Model file for the job. Use its own axes, mm. Face numbers are marked on the shaded views. Coordinates: 2 decimals unless noted, no trailing zeros. Write each loop counter-clockwise with the first axis right and the second up, starting at its lowest first coordinate (ties: lowest second). Pieces come first, ordered by that corner, then holes. Notation, with made-up numbers: (78.25, 63) - (137.25, 63) arc R22 cw to (137.25, 101) - close; hole circle Ø6 at (-8, -38). An arc over 180 degrees is marked (long way). Put each result on its own line as item: value. Start each with the question number.
1. Saw through at D-D, the plane x = 66. Write the cut outline in (y, z).
2. Pull direction X, two halves, no side cores. Call the marked faces 1, 2 and 3: released by +X, released by -X, zero draft, split by the parting line, or undercut.
3. Drill centre lines: L1, parallel to X at y = 7, z = -11; L2, parallel to X at y = 29, z = -8; L3, parallel to Z at x = 21, y = 13. Where is each one in solid material? Low to high. Write a range as from..to.
4. Drop a flat-ended pin along its axis: P1, Ø4, axis at x = -52.5, y = 15, coming from the -Z side. Give the stop position or say it passes through.
5. Saw through at A-A, the plane z = 15. Write the cut outline in (x, y).
6. Saw through at B-B, the plane x = -7. Write the cut outline in (y, z).
7. Saw through at C-C, the plane y = 8.5. Write the cut outline in (x, z), plus the area to 4 significant figures.
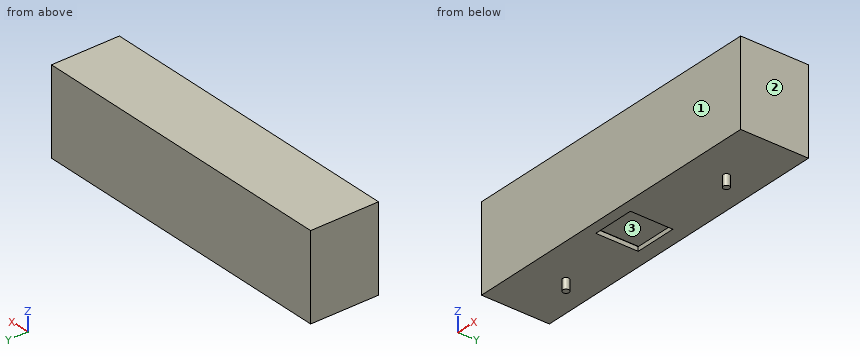
```python
from build123d import *

# Parameters (mm, degrees)
SKETCH1_W           = 150
SKETCH1_H           = 40
BOSS_EXTRUDE1_DEPTH = 30
SHELL3_T            = -2
SKETCH3_W           = 20
SKETCH3_H           = 20
CUT_EXTRUDE1_DEPTH  = 5
SKETCH6_W           = 19.798687527
SKETCH6_H           = 12.601964569
BOSS_EXTRUDE3_DEPTH = 24
SKETCH7_W           = 150
SKETCH7_H           = 40
BOSS_EXTRUDE4_DEPTH = 2
SKETCH8_R           = 1.5
BOSS_EXTRUDE5_DEPTH = 5
SKETCH9_R           = 1.5
BOSS_EXTRUDE6_DEPTH = 5


with BuildPart() as part:
    # Sketch1 → Boss-Extrude1 (new body)
    with BuildSketch(Plane(origin=(0, 0, 0), x_dir=(1, 0, 0), z_dir=(0, 1, 0))):
        Rectangle(SKETCH1_W, SKETCH1_H)
    extrude(amount=BOSS_EXTRUDE1_DEPTH)

    # Shell3
    shell3_openings = [part.faces().sort_by_distance(p)[0] for p in [
        (0, 30, 0),
    ]]
    offset(amount=SHELL3_T, openings=shell3_openings, kind=Kind.INTERSECTION)

    # Sketch3 → Cut-Extrude1 (cut)
    with BuildSketch(Plane(origin=(0, 0, -20), x_dir=(-1, 0, 0), z_dir=(0, 0, -1))):
        with Locations((4.963499303, 15)):
            Rectangle(SKETCH3_W, SKETCH3_H)
    extrude(amount=-CUT_EXTRUDE1_DEPTH, mode=Mode.SUBTRACT)

    # Sketch6 → Boss-Extrude3 (add)
    with BuildSketch(Plane(origin=(0, 2, 0), x_dir=(1, 0, 0), z_dir=(0, 1, 0))):
        with Locations((-4.895398538, 11.699017716)):
            Rectangle(SKETCH6_W, SKETCH6_H)
    extrude(amount=BOSS_EXTRUDE3_DEPTH)

    # Sketch7 → Boss-Extrude4 (add)
    with BuildSketch(Plane(origin=(0, 30, 0), x_dir=(1, 0, 0), z_dir=(0, 1, 0))):
        Rectangle(SKETCH7_W, SKETCH7_H)
    extrude(amount=BOSS_EXTRUDE4_DEPTH)

    # Sketch8 → Boss-Extrude5 (add)
    with BuildSketch(Plane(origin=(0, 0, -20), x_dir=(-1, 0, 0), z_dir=(0, 0, -1))):
        with Locations(Location((-46.510205531, 16.504268765, 0), (0, 0, 180))):
            Circle(SKETCH8_R)
    extrude(amount=BOSS_EXTRUDE5_DEPTH)

    # Sketch9 → Boss-Extrude6 (add)
    with BuildSketch(Plane(origin=(0, 0, -20), x_dir=(-1, 0, 0), z_dir=(0, 0, -1))):
        with Locations(Location((47, 17.020870221, 0), (0, 0, 180))):
            Circle(SKETCH9_R)
    extrude(amount=BOSS_EXTRUDE6_DEPTH)


solid = part.part
```
Final values:
1. outline: (0, -20) - (32, -20) - (32, 20) - (0, 20) - close; hole (2, -18) - (30, -18) - (30, 18) - (2, 18) - close
2. face 1: zero draft
2. face 2: released by +X
2. face 3: undercut
3. L1: x = -75..-73, -14.79..5, 73..75
3. L2: x = -75..-73, 73..75
3. L3: z = -20..-18, 18..20
4. P1: stops at z = -20
5. outline: (-75, 0) - (75, 0) - (75, 32) - (-75, 32) - close; hole (-73, 2) - (73, 2) - (73, 30) - (-73, 30) - close
6. outline: (0, -20) - (5, -20) - (5, -18) - (25, -18) - (25, -20) - (32, -20) - (32, 20) - (0, 20) - close; hole (2, -5.4) - (26, -5.4) - (26, -18) - (30, -18) - (30, 18) - (2, 18) - close
7. outline: (-75, -20) - (-14.96, -20) - (-14.96, -18) - (-73, -18) - (-73, 18) - (73, 18) - (73, -18) - (5.04, -18) - (5.04, -20) - (75, -20) - (75, 20) - (-75, 20) - close; (-14.79, -18) - (5, -18) - (5, -5.4) - (-14.79, -5.4) - close
7. area: 953.5 mm²
